Input: part model. Units: mm. Frame: model coordinates. Face numbers are marked on the shaded views. Round coordinates to 2 decimals unless told otherwise and drop trailing zeros. Loops run counter-clockwise (first coordinate to the right, second up) from the corner with the lowest first, then second, coordinate; pieces in that order, holes last. Notation, with made-up numbers: (83.5, 49) - (92.5, 49) arc R19 ccw to (92.5, 62) - close; hole circle Ø2 at (-19, 8). An arc over 180 degrees is marked (long way). Use CSV: the item, a comma, the result in double quotes. Start each with the question number.
1. Cut plane D-D (x = 2). Return loops of the section in (y, z), and give its area (3 significant figures).
2. Pull-direction query (Z, two-part tool) for the marked faces 1, 2, 3 and 4; classes: +Z half, -Z half, draft (parallel to the pull), parting line (faces both ways), or undercut.
3. Pin query (flat end, axial travel): P1, Ø2.5, axis at x = -9, y = 0, coming from the -Z side; P2, Ø3.5, axis at x = 7, y = 1.5, coming from the -Z side; P3, Ø3, axis at x = 3.5, z = 116.5, coming from the +Y side. Return the tip coordinate at first contact, or that it passes through.
4. Cut plane C-C (z = 86.5). Return loops of the section in (x, y).
5. Material intervals for probe 1 along Z at (x, y) = (0.5, 5.25); probe 2 along X at (y, z) = (-3.25, 51); probe 3 along Y at (x, z) = (-11, 125.5), sorted ascending. Write a range as from..to.
6. Cut plane A-A (x = -9). Return loops of the section in (y, z).
7. Cut plane B-B (y = 0). Return loops of the section in (x, z), and give its area (3 significant figures).
```python
from build123d import *

# Parameters (mm, degrees)
F0_W     = 37
F0_H     = 15
F1_DEPTH = 150
F2_W     = 31
F2_H     = 144
F3_DEPTH = 12
F4_R     = 2
F5_DEPTH = 150.001
F6_R     = 1
F7_R     = 1


with BuildPart() as f1:
    # F0 (on Top) → F1 (new body)
    with BuildSketch(Plane.XY):
        Rectangle(F0_W, F0_H)
    extrude(amount=F1_DEPTH)

    # F2 (on face) → F3 (cut)
    with BuildSketch(Plane(origin=(0, 7.5, 0), x_dir=(-1, 0, 0), z_dir=(0, 1, 0))):
        with Locations((0, 75)):
            Rectangle(F2_W, F2_H)
    extrude(amount=-F3_DEPTH, mode=Mode.SUBTRACT)

    # F4 (on face) → F5 (cut, through all)
    with BuildSketch(Plane.XY.offset(150)):
        with Locations((9, 0)):
            Circle(F4_R)
        with Locations((-9, 0)):
            Circle(F4_R)
    extrude(amount=-F5_DEPTH, mode=Mode.SUBTRACT)

    # F6
    f6_edges = [f1.edges().sort_by_distance(p)[0] for p in [
        (-18.5, 0, 150),
        (18.5, 0, 150),
        (-18.5, 0, 0),
        (18.5, 0, 0),
    ]]
    fillet(f6_edges, radius=F6_R)

    # F7
    f7_edges = [f1.edges().sort_by_distance(p)[0] for p in [
        (18.5, -7.5, 75),
        (18.5, 7.5, 75),
    ]]
    fillet(f7_edges, radius=F7_R)


solid = f1.part
```
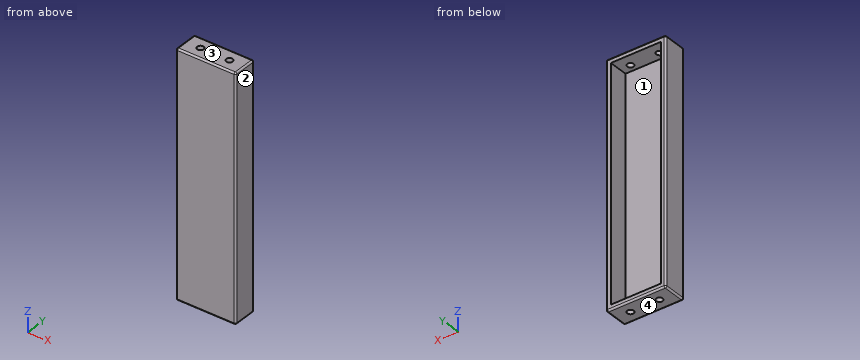
Established:
1,outline,"(-7.5, 1) arc R1 ccw to (-6.5, 0) - (6.5, 0) arc R1 ccw to (7.5, 1) - (7.5, 3) - (-4.5, 3) - (-4.5, 147) - (7.5, 147) - (7.5, 149) arc R1 ccw to (6.5, 150) - (-6.5, 150) arc R1 ccw to (-7.5, 149) - close"
1,area,"521 mm2"
2,face 1,"undercut"
2,face 2,"draft"
2,face 3,"+Z half"
2,face 4,"-Z half"
3,P1,"passes through"
3,P2,"stops at z = 0"
3,P3,"stops at y = -4.5"
4,outline,"(-18.5, -6.5) arc R1 ccw to (-17.5, -7.5) - (17.5, -7.5) arc R1 ccw to (18.5, -6.5) - (18.5, 6.5) arc R1 ccw to (17.5, 7.5) - (15.5, 7.5) - (15.5, -4.5) - (-15.5, -4.5) - (-15.5, 7.5) - (-17.5, 7.5) arc R1 ccw to (-18.5, 6.5) - close"
5,probe 1,"z = 0..3, 147..150"
5,probe 2,"x = -18.5..-15.5, 15.5..18.5"
5,probe 3,"y = -7.5..-4.5"
6,outline,"(-7.5, 1) arc R1 ccw to (-6.5, 0) - (-2, 0) - (-2, 3) - (-4.5, 3) - (-4.5, 147) - (-2, 147) - (-2, 150) - (-6.5, 150) arc R1 ccw to (-7.5, 149) - close; (2, 0) - (6.5, 0) arc R1 ccw to (7.5, 1) - (7.5, 3) - (2, 3) - close; (2, 147) - (7.5, 147) - (7.5, 149) arc R1 ccw to (6.5, 150) - (2, 150) - close"
7,outline,"(-18.5, 1) arc R1 ccw to (-17.5, 0) - (-11, 0) - (-11, 3) - (-15.5, 3) - (-15.5, 147) - (-11, 147) - (-11, 150) - (-17.5, 150) arc R1 ccw to (-18.5, 149) - close; (-7, 0) - (7, 0) - (7, 3) - (-7, 3) - close; (-7, 147) - (7, 147) - (7, 150) - (-7, 150) - close; (11, 0) - (17.5, 0) arc R1 ccw to (18.5, 1) - (18.5, 149) arc R1 ccw to (17.5, 150) - (11, 150) - (11, 147) - (15.5, 147) - (15.5, 3) - (11, 3) - close"
7,area,"1,040 mm2"
